The model under review builds one solid part; all positions refer to its coordinate system, in mm. Face numbers are marked on the shaded views. A direction names the side the tool comes from. Round coordinates to 2 decimals unless told otherwise and drop trailing zeros. Loops run counter-clockwise (first coordinate to the right, second up) from the corner with the lowest first, then second, coordinate; pieces in that order, holes last. Notation, with made-up numbers: (24.5, -18) -> (43.5, -18) arc R13 ccw to (43.5, -6) -> close; hole circle Ø1 at (-1.5, -7.5). An arc over 180 degrees is marked (long way). Write each question's results on one line, items separated by ' | '. Start each with the question number.
Item 1: Tool access review of the marked faces 1 and 2: name each direction out of +Z, -Z, +X, -X, +Y, -Y from which nothing blocks a thin tool from reaching the whole face with its end or side.
Item 2: Mouldability with a two-part tool opening along Y and no side actions: class the marked faces 3, 4, 5 and 6 as pulls with the +Y half, pulls with the -Y half, needs draft (parallel to the pull), parting line crosses it, or undercut.
Item 3: We need section A-A (y = 0). Give the boundary of the cut face in (x, z), and give its area (3 significant figures).
Item 4: Clearance check with a flat-ended pin moving along its axis: pin 1 Ø1 at (x, y) = (3, 0) entering from +Z. State where the tip first meets the part, or that it passes through.
Item 5: We need section C-C (z = 4.5). Give the boundary of the cut face in (x, y).
Item 6: We need section B-B (z = 2.5). Give the boundary of the cut face in (x, y).
Item 7: We need section D-D (x = -1.5). Give the boundary of the cut face in (y, z).
Item 8: For L1, parallel to X at y = 8.25, z = 2.5; L2, parallel to Y at x = -1, z = 0.5; L3, parallel to Z at x = 1, y = -5.5, list the stretches that pass through material, from the lowest coordinate up. Write a range as from..to.
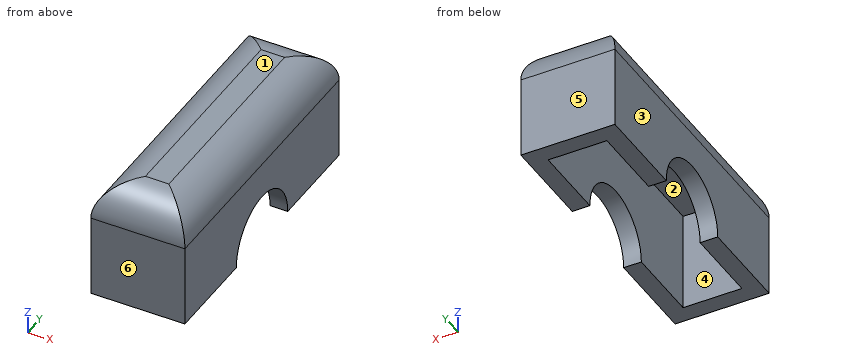
from build123d import *

# Parameters (mm, degrees)
F0_W     = 8
F0_H     = 24
F1_DEPTH = 10
F2_T     = -1.5
F4_D     = 8
F5_R     = 3


with BuildPart() as f1:
    # F0 (on Top) → F1 (new body)
    with BuildSketch(Plane.XY):
        Rectangle(F0_W, F0_H)
    extrude(amount=F1_DEPTH)

    # F2
    f2_openings = [f1.faces().sort_by_distance(p)[0] for p in [
        (0, 0, 0),
    ]]
    offset(amount=F2_T, openings=f2_openings)

    # F4 (through all)
    with Locations(Plane.YZ.offset(4)):
        with Locations((0, 0)):
            Hole(F4_D / 2)

    # F5
    f5_edges = [f1.edges().sort_by_distance(p)[0] for p in [
        (0, -12, 10),
        (4, 0, 10),
        (0, 12, 10),
        (-4, 0, 10),
    ]]
    fillet(f5_edges, radius=F5_R)


solid = f1.part
Here are the results:
1) face 1: +Z, +X, -X, +Y, -Y | face 2: -Z
2) face 3: needs draft | face 4: undercut | face 5: pulls with the +Y half | face 6: pulls with the -Y half
3) outline: (-4, 4) -> (-2.5, 4) -> (-2.5, 8.5) -> (2.5, 8.5) -> (2.5, 4) -> (4, 4) -> (4, 7) arc R3 ccw to (1, 10) -> (-1, 10) arc R3 ccw to (-4, 7) -> close | area: 21.6 mm2
4) pin 1: stops at z = 9.6
5) outline: (-4, -12) -> (4, -12) -> (4, 12) -> (-4, 12) -> close; hole (-2.5, -10.5) -> (2.5, -10.5) -> (2.5, 10.5) -> (-2.5, 10.5) -> close
6) outline: (-4, -12) -> (4, -12) -> (4, -3.12) -> (2.5, -3.12) -> (2.5, -10.5) -> (-2.5, -10.5) -> (-2.5, -3.12) -> (-4, -3.12) -> close; (-4, 3.12) -> (-2.5, 3.12) -> (-2.5, 10.5) -> (2.5, 10.5) -> (2.5, 3.12) -> (4, 3.12) -> (4, 12) -> (-4, 12) -> close
7) outline: (-12, 0) -> (-10.5, 0) -> (-10.5, 8.5) -> (10.5, 8.5) -> (10.5, 0) -> (12, 0) -> (12, 7) arc R3 ccw to (9.5, 9.96) -> (-9.5, 9.96) arc R3 ccw to (-12, 7) -> close
8) L1: x = -4..-2.5, 2.5..4 | L2: y = -12..-10.5, 10.5..12 | L3: z = 8.5..10
